For this review, take the finished solid that the model builds, in its own axes (mm). A direction names the side the tool comes from. Round coordinates to 2 decimals unless told otherwise and drop trailing zeros. Order: outer loops, then holes, each group sorted by start corner. A loop starts at its lowest first (then second) coordinate and runs counter-clockwise, first axis right, second up. Notation, with made-up numbers: M 86,42.5 L 118,42.5 A30 ccw 118,70.5 Z; hole C 13.25,-27 d11. An arc over 180 degrees is marked long. Answer as a JSON object with one key per item and string values.
from build123d import *

# Parameters (mm, degrees)
SKETCH1_R           = 3
BOSS_EXTRUDE1_DEPTH = 3
SKETCH2_R           = 2
BOSS_EXTRUDE2_DEPTH = 8
SKETCH3_R           = 1.5
BOSS_EXTRUDE3_DEPTH = 4
CUT_EXTRUDE1_DEPTH  = 2
CHAMFER1_SIZE       = 0.25


with BuildPart() as part:
    # Sketch1 → Boss-Extrude1 (new body)
    with BuildSketch(Plane(origin=(0, 0, 0), x_dir=(1, 0, 0), z_dir=(0, 1, 0))):
        with Locations(Location((0, 0, 0), (0, 0, 270))):
            Circle(SKETCH1_R)
    extrude(amount=BOSS_EXTRUDE1_DEPTH)

    # Sketch2 → Boss-Extrude2 (add)
    with BuildSketch(Plane.XZ):
        with Locations(Location((0, 0, 0), (0, 0, 90))):
            Circle(SKETCH2_R)
    extrude(amount=BOSS_EXTRUDE2_DEPTH)

    # Sketch3 → Boss-Extrude3 (add)
    with BuildSketch(Plane.XZ.offset(8)):
        with Locations(Location((0, 0, 0), (0, 0, 270))):
            Circle(SKETCH3_R)
    extrude(amount=BOSS_EXTRUDE3_DEPTH)

    # Sketch4 → Cut-Extrude1 (cut)
    with BuildSketch(Plane(origin=(0, 3, 0), x_dir=(1, 0, 0), z_dir=(0, 1, 0))):
        Polygon((0.577350269, 1), (-0.577350269, 1), (-1.154700538, 0), (-0.577350269, -1), (0.577350269, -1), (1.154700538, 0), align=None)
    extrude(amount=-CUT_EXTRUDE1_DEPTH, mode=Mode.SUBTRACT)

    # Chamfer1
    chamfer1_edges = [part.edges().sort_by_distance(p)[0] for p in [
        (0, 3, -3),
    ]]
    chamfer(chamfer1_edges, length=CHAMFER1_SIZE)


solid = part.part
1) Add section A-A on x = 0. State the section outline as (y, z) points.
Geometry check:
{"outline": "M -12,-1.5 L -8,-1.5 L -8,-2 L 0,-2 L 0,-3 L 2.75,-3 L 3,-2.75 L 3,-1 L 1,-1 L 1,1 L 3,1 L 3,2.75 L 2.75,3 L 0,3 L 0,2 L -8,2 L -8,1.5 L -12,1.5 Z"}
2) Add section C-C on y = -4. State the section outline as (x, z) points, and give its area (3 significant figures).
Geometry check:
{"outline": "C 0,0 d4", "area": "12.6 mm²"}
3) For L1, parallel to Y at x = 1.8, z = 1; L2, parallel to Y at x = -1.9, z = 0.05; L3, parallel to Z at x = 1.2, y = 1, list the stretches that pass through material, from the lowest coordinate up.
Geometry check:
{"L1": "y = 0 to 3", "L2": "y = -8 to 3", "L3": "z = -2.75 to 2.75"}
4) Machinability: for faces 4 (the flat face through (0, 3, 1.2)), 5 (the cylindrical face through (2, -4, 0)), 6 (the flat face through (0, 2, -1)), which of the approach directions +Z, -Z, +X, -X, +Y, -Y give a long, thin tool a straight path to every point of the face, cutting with its end or side? Answer none if there is none.
Geometry check:
{"face 4": "+Z, -Z, +X, -X, +Y", "face 5": "-Y", "face 6": "+Y"}
5) Insertion check: P1, Ø1, axis at x = 0.5, z = -0.5, coming from the +Y side; P2, Ø3, axis at x = 1.5, y = -10, coming from the +Z side; P3, Ø0.6, axis at x = 0.5, y = 1.5, coming from the -Z side. Each pin has a flat end and moves straight along its axis. Give the tip position at first contact, or say it passes through.
Geometry check:
{"P1": "stops at y = 3", "P2": "stops at z = 1.5", "P3": "stops at z = -2.99"}
6) Mouldability with a two-part tool opening along X and no side actions: class faces 1 (the cylindrical face through (0.45, -9.97, -1.43)), 2 (the flat face through (-1, 0, 2)), 3 (the flat face through (0, 1, 0)) as +X half, -X half, draft (parallel to the pull), parting line (faces both ways), or undercut.
Geometry check:
{"face 1": "parting line", "face 2": "draft", "face 3": "undercut"}
7) Add section B-B on y = -9.75. State the section outline as (x, z) points, and give its area (3 significant figures).
Geometry check:
{"outline": "C 0,0 d3", "area": "7.07 mm²"}
